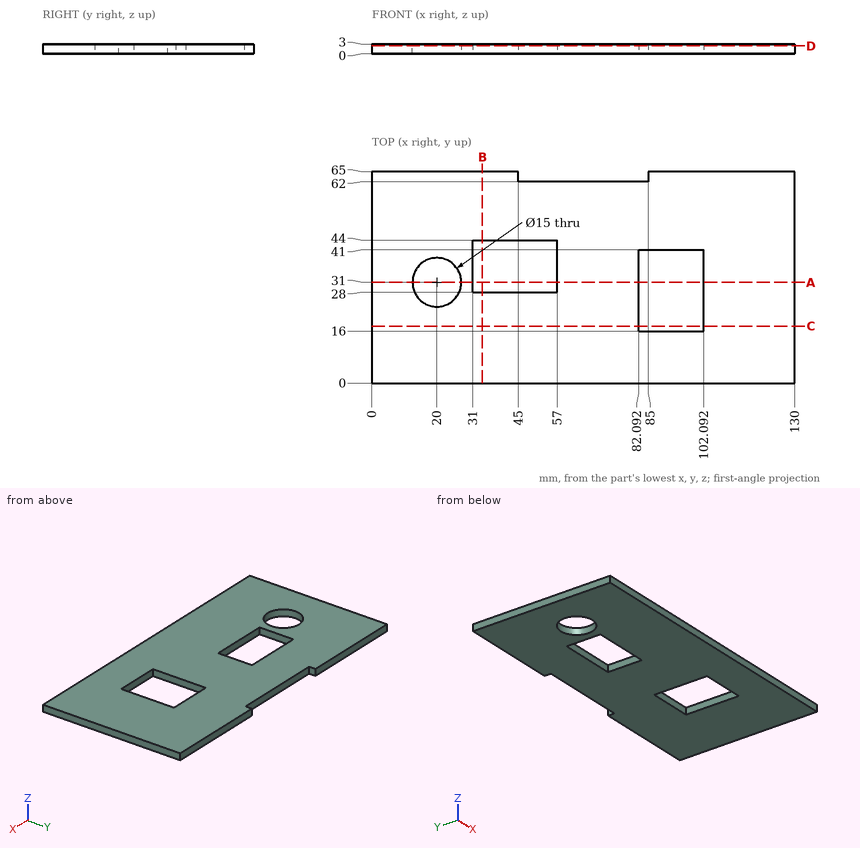
Can you work these out from the drawing? Everything is in mm from the part's minimum corner. Give positions to 0.01 mm unless a question says otherwise; leave off trailing zeros. Loops run counter-clockwise (first coordinate to the right, second up) from the corner with the lowest first, then second, coordinate; pieces in that order, holes last. Notation, with made-up numbers: (49, 24.25) - (71, 24.25) arc R20 cw to (71, 40.25) - close; hole circle Ø7 at (41, 58.5). An arc over 180 degrees is marked (long way). Use one line per item in the form item = value.
1. I want a section at A-A (y = 31). Please give me the cut outline in (x, z).
Response values:
outline = (0, 0) - (12.5, 0) - (12.5, 3) - (0, 3) - close; (27.5, 0) - (31, 0) - (31, 3) - (27.5, 3) - close; (57, 0) - (82.09, 0) - (82.09, 3) - (57, 3) - close; (102.09, 0) - (130, 0) - (130, 3) - (102.09, 3) - close
2. I want a section at D-D (z = 2.4). Please give me the cut outline in (x, y).
Response values:
outline = (0, 0) - (130, 0) - (130, 65) - (85, 65) - (85, 62) - (45, 62) - (45, 65) - (0, 65) - close; hole circle Ø15 at (20, 31); hole (31, 28) - (57, 28) - (57, 44) - (31, 44) - close; hole (82.09, 16) - (102.09, 16) - (102.09, 41) - (82.09, 41) - close
3. I want a section at C-C (y = 17.5). Please give me the cut outline in (x, z), and give its area (3 significant figures).
Response values:
outline = (0, 0) - (82.09, 0) - (82.09, 3) - (0, 3) - close; (102.09, 0) - (130, 0) - (130, 3) - (102.09, 3) - close
area = 330 mm²
4. I need wall thicknesses on probe 1 along X at (y, z) = (17, 2.25); probe 2 along Y at (x, z) = (20, 1.7); probe 3 along Y at (x, z) = (42, 1.7). Which ranges of each line are inside material? Lowest first, please.
Response values:
probe_1 = 0 to 82.09, 102.09 to 130
probe_2 = 0 to 23.5, 38.5 to 65
probe_3 = 0 to 28, 44 to 65
5. I'm going to push a flat-ended pin straight in: pin 1 Ø1.5 at (x, z) = (58.5, 1) entering from +Y. Where does the tip first touch, or does it pass through?
Response values:
pin_1 = 62
6. I want a section at B-B (x = 34). Please give me the cut outline in (y, z), and give its area (3 significant figures).
Response values:
outline = (0, 0) - (28, 0) - (28, 3) - (0, 3) - close; (44, 0) - (65, 0) - (65, 3) - (44, 3) - close
area = 147 mm²
